Verification items for this drawing (mm, ordinates from the low corner). A direction names the side the tool comes from. Round coordinates to 2 decimals unless told otherwise and drop trailing zeros. Loops run counter-clockwise (first coordinate to the right, second up) from the corner with the lowest first, then second, coordinate; pieces in that order, holes last. Notation, with made-up numbers: (-10.75, 76.5) - (42.25, 76.5) arc R31 ccw to (42.25, 107.5) - close; hole circle Ø9 at (-34.5, 58). An arc over 180 degrees is marked (long way). Use a Markdown table: item, result. Add a question column.
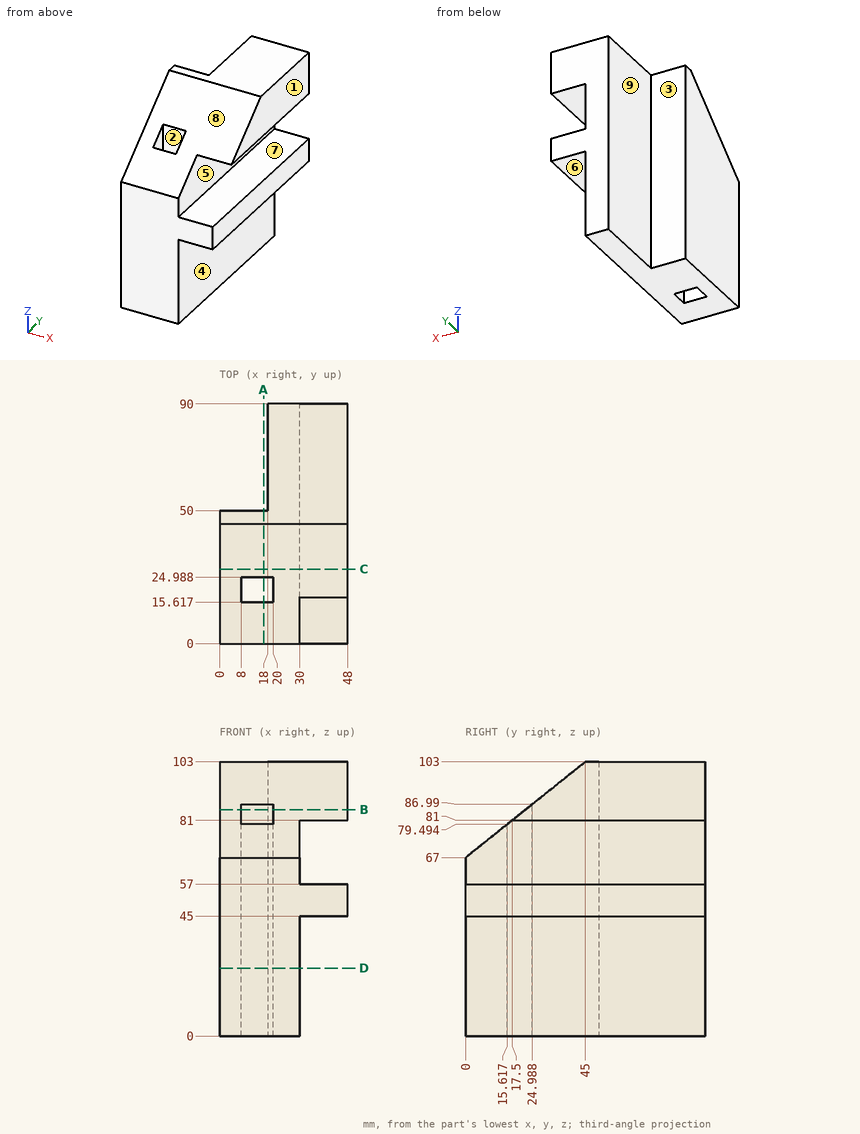
Q1. Thickness scan on line 1 along Z through (x, y) = (46.5, 84.5); line 2 along X through (y, z) = (21.5, 31); line 3 along Y through (x, z) = (19.5, 33.5). Record the ranges inside material, lowest first.
Q2. Section check D-D on z = 25.5. Record the cut outline in (x, y), plus the area to 3 significant figures.
Q3. Section check B-B on z = 85. Record the cut outline in (x, y), plus the area to 3 significant figures.
Q4. Go/stop test with flat-tipped pins: pin 1 Ø5 at (x, z) = (18, 82.5) entering from -Y; pin 2 Ø2 at (y, z) = (64, 60.5) entering from -X; pin 3 Ø14.5 at (x, y) = (40.5, 60.5) entering from -Z. Record where each tip stops, or that it passes through.
Q5. Section check A-A on x = 16.5. Record the cut outline in (y, z), plus the area to 3 significant figures.
Q6. Section check C-C on y = 28. Record the cut outline in (x, z).
Q7. Set-up check for the marked faces 1, 2, 3, 4 and 5: record each of +Z, -Z, +X, -X, +Y, -Y from which the full face is reachable in a straight line by a thin tool's end or side.
Q8. Release check for a two-part mould opening along Z. For the marked faces 6, 7, 8 and 9 record: +Z half, -Z half, draft (parallel to the pull), parting line (faces both ways), or undercut.
Determined:
| question | item | result |
|---|---|---|
| 1 | line 1 | z = 45 to 57, 81 to 103 |
| 1 | line 2 | x = 0 to 8, 20 to 30 |
| 1 | line 3 | y = 0 to 15.62, 24.99 to 90 |
| 2 | outline | (0, 0) - (30, 0) - (30, 90) - (18, 90) - (18, 50) - (0, 50) - close; hole (8, 15.62) - (20, 15.62) - (20, 24.99) - (8, 24.99) - close |
| 2 | area | 1,870 mm² |
| 3 | outline | (0, 22.5) - (8, 22.5) - (8, 24.99) - (20, 24.99) - (20, 22.5) - (48, 22.5) - (48, 90) - (18, 90) - (18, 50) - (0, 50) - close |
| 3 | area | 2,490 mm² |
| 4 | pin 1 | stops at y = 17.5 |
| 4 | pin 2 | stops at x = 18 |
| 4 | pin 3 | stops at z = 45 |
| 5 | outline | (0, 0) - (15.62, 0) - (15.62, 79.49) - (0, 67) - close; (24.99, 0) - (50, 0) - (50, 103) - (45, 103) - (24.99, 86.99) - close |
| 5 | area | 3,560 mm² |
| 6 | outline | (0, 0) - (30, 0) - (30, 45) - (48, 45) - (48, 57) - (30, 57) - (30, 81) - (48, 81) - (48, 89.4) - (0, 89.4) - close |
| 7 | face 1 | +Z, -Z, +X, +Y, -Y |
| 7 | face 2 | +Z, -Z |
| 7 | face 3 | +Z, -Z, -X, +Y |
| 7 | face 4 | -Z, +X, +Y, -Y |
| 7 | face 5 | +X, +Y, -Y |
| 8 | face 6 | -Z half |
| 8 | face 7 | undercut |
| 8 | face 8 | +Z half |
| 8 | face 9 | draft |
